from build123d import *

# Parameters (mm, degrees)
ESQUISSE1_R        = 3.75
ESQUISSE1_W        = 12.12
ESQUISSE1_H        = 28.68
BOSS_EXTRU_1_DEPTH = 3
CONG_3_R           = 1


with BuildPart() as part:
    # Esquisse1 → Boss.-Extru.1 (new body)
    with BuildSketch(Plane.XY):
        Polygon((-30, 37.5), (30, 37.5), (30, 27.5), (24, 27.5), (24, 29), (21, 29), (21, 27.5), (16, 27.5), (16, 24.25), (21, 24.25), (21, 22.75), (24, 22.75), (24, 24.25), (30, 24.25), (30, 12.5), (30, -12.5), (35, -12.5), (35, -27.5), (30, -27.5), (30, -37.5), (-30, -37.5), (-30, -27.5), (-24, -27.5), (-24, -29), (-21, -29), (-21, -27.5), (-16, -27.5), (-16, -24.25), (-21, -24.25), (-21, -22.75), (-24, -22.75), (-24, -24.25), (-30, -24.25), (-30, -12.5), (-30, 12.5), (-30, 24.25), (-24, 24.25), (-24, 22.75), (-21, 22.75), (-21, 24.25), (-16, 24.25), (-16, 27.5), (-21, 27.5), (-21, 29), (-24, 29), (-24, 27.5), (-30, 27.5), align=None)
        Circle(ESQUISSE1_R, mode=Mode.SUBTRACT)
        with Locations((15, -1.66)):
            Rectangle(ESQUISSE1_W, ESQUISSE1_H, mode=Mode.SUBTRACT)
    extrude(amount=BOSS_EXTRU_1_DEPTH)

    # Congé3
    cong_3_edges = [part.edges().sort_by_distance(p)[0] for p in [
        (35, -12.5, 1.5),
        (35, -27.5, 1.5),
    ]]
    fillet(cong_3_edges, radius=CONG_3_R)


solid = part.part
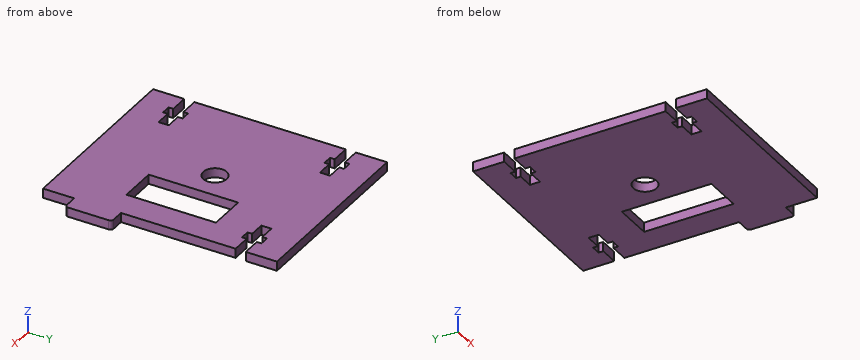
For this review, take the finished solid that the model builds, in its own axes (mm). Coordinates: 2 decimals unless noted, no trailing zeros. Loops run counter-clockwise (first coordinate to the right, second up) from the corner with the lowest first, then second, coordinate; pieces in that order, holes last. Notation, with made-up numbers: (-35, 40.25) - (12, 40.25) arc R19 ccw to (12, 66.25) - close; hole circle Ø9 at (-25.75, 10). An arc over 180 degrees is marked (long way). Return JSON: item names as keys, results as strings.
Item 1: For line 1 (Y direction, x = -27, z = 2.3); line 2 (Y direction, x = 17.5, z = 2.2); line 3 (Y direction, x = 0, z = 1.6), list the stretches that pass through material, from the lowest coordinate up.
Determined:
{"line 1": "y = -37.5 to -27.5, -24.25 to 24.25, 27.5 to 37.5", "line 2": "y = -37.5 to -16, 12.68 to 24.25, 27.5 to 37.5", "line 3": "y = -37.5 to -3.75, 3.75 to 37.5"}
Item 2: Take a section at B-B (x = 0). Give the boundary of the cut face in (y, z), then the cut area to 4 significant figures.
Determined:
{"outline": "(-37.5, 0) - (-3.75, 0) - (-3.75, 3) - (-37.5, 3) - close; (3.75, 0) - (37.5, 0) - (37.5, 3) - (3.75, 3) - close", "area": "202.5 mm2"}
Item 3: Take a section at A-A (y = 8.5). Give the boundary of the cut face in (x, z).
Determined:
{"outline": "(-30, 0) - (8.94, 0) - (8.94, 3) - (-30, 3) - close; (21.06, 0) - (30, 0) - (30, 3) - (21.06, 3) - close"}
Item 4: Insertion check: pin 1 (0.9 mm diameter, centred on y = 25.5, z = 1.5, fed in from -X); pin 2 (0.9 mm diameter, centred on x = 32.5, z = 2, fed in from +Y); pin 3 (0.9 mm diameter, centred on y = 14, z = 1, fed in from +X). Each pin has a flat end and moves straight along its axis. Give the tip position at first contact, or say it passes through.
Determined:
{"pin 1": "stops at x = -16", "pin 2": "stops at y = -12.5", "pin 3": "stops at x = 30"}
Item 5: Take a section at C-C (y = 0). Give the boundary of the cut face in (x, z).
Determined:
{"outline": "(-30, 0) - (-3.75, 0) - (-3.75, 3) - (-30, 3) - close; (3.75, 0) - (8.94, 0) - (8.94, 3) - (3.75, 3) - close; (21.06, 0) - (30, 0) - (30, 3) - (21.06, 3) - close"}
Item 6: Take a section at D-D (z = 0.6). State how many separate pieces and enclosed holes the cut face has, then the cut area to 3 significant figures.
Determined:
{"separate pieces": "1", "enclosed holes": "2", "area": "4,020 mm2"}
